from build123d import *

# Parameters (mm, degrees)
F1_DEPTH = 6


with BuildPart() as f1:
    # F0 (on Front) → F1 (new body)
    with BuildSketch(Plane.XZ):
        with BuildLine():
            Line((100, 60), (0, 60))
            Line((0, 60), (0, -60))
            Line((0, -60), (100, -60))
            Line((100, -60), (100, -40))
            Line((100, -40), (30, -40))
            ThreePointArc((30, -40), (22.928932, -37.071068), (20, -30))
            Line((20, -30), (20, 37))
            ThreePointArc((20, 37), (20.87868, 39.12132), (23, 40))
            Line((23, 40), (100, 40))
            Line((100, 40), (100, 60))
        make_face()
    extrude(amount=F1_DEPTH)


solid = f1.part
The listing builds one solid part. Answer for the finished solid, in the listing's coordinates (mm). A direction names the side the tool comes from. Give positions to 0.01 mm unless a question says otherwise; leave off trailing zeros. Write each loop counter-clockwise with the first axis right and the second up, starting at its lowest first coordinate (ties: lowest second). Pieces come first, ordered by that corner, then holes. Notation, with made-up numbers: (37.25, -2) -> (70.25, -2) arc R29 cw to (70.25, 22) -> close; hole circle Ø1 at (75, -29). An arc over 180 degrees is marked (long way). One line per question, with ' | ' between items. Start each with the question number.
1. For faces 4 (the flat face through (61, -3, 40)), 5 (the flat face through (100, -3, -50)), determine the directions among +Z, -Z, +X, -X, +Y, -Y from which every point of the face is accessible in a straight line to the end or side of a thin tool.
2. Find the intervals of material crossed by probe 1 along Z at (x, y) = (93, -4.8); probe 2 along X at (y, z) = (-2.1, -17.5); probe 3 along Z at (x, y) = (24, -2.2), in increasing order.
3. Section A-A (x = 55.5) is taken. Determine the outline of the cut face in (y, z), plus the area to 3 significant figures.
4. Section C-C (x = 26.5) is taken. Determine the outline of the cut face in (y, z), plus the area to 3 significant figures.
5. For a pull along Z with two mould halves and no side action, classify faces 1 (the flat face through (65, -3, -40)), 2 (the flat face through (49, -3, -60)), 3 (the flat face through (16, 0, 14)) as pulls with the +Z half, pulls with the -Z half, needs draft (parallel to the pull), parting line crosses it, or undercut.
6. Section D-D (z = 24) is taken. Determine the outline of the cut face in (x, y).
7. Section B-B (y = -4.7) is taken. Determine the outline of the cut face in (x, z), plus the area to 3 significant figures.
Response values:
1) face 4: +X, +Y, -Y | face 5: +Z, -Z, +X, +Y, -Y
2) probe 1: -60 to -40, 40 to 60 | probe 2: 0 to 20 | probe 3: -60 to -38, 40 to 60
3) outline: (-6, -60) -> (0, -60) -> (0, -40) -> (-6, -40) -> close; (-6, 40) -> (0, 40) -> (0, 60) -> (-6, 60) -> close | area: 240 mm2
4) outline: (-6, -60) -> (0, -60) -> (0, -39.37) -> (-6, -39.37) -> close; (-6, 40) -> (0, 40) -> (0, 60) -> (-6, 60) -> close | area: 244 mm2
5) face 1: undercut | face 2: pulls with the -Z half | face 3: needs draft
6) outline: (0, -6) -> (20, -6) -> (20, 0) -> (0, 0) -> close
7) outline: (0, -60) -> (100, -60) -> (100, -40) -> (30, -40) arc R10 cw to (20, -30) -> (20, 37) arc R3 cw to (23, 40) -> (100, 40) -> (100, 60) -> (0, 60) -> close | area: 5,620 mm2
